Read the model definition and answer for the solid it produces. Units are mm, in the model's axes. Round coordinates to 2 decimals unless told otherwise and drop trailing zeros. Write each loop counter-clockwise with the first axis right and the second up, starting at its lowest first coordinate (ties: lowest second). Pieces come first, ordered by that corner, then holes. Notation, with made-up numbers: (57.25, 35) - (116.25, 35) arc R33 ccw to (116.25, 69) - close; hole circle Ø11 at (-8, 9.25). An arc over 180 degrees is marked (long way). Use one line per item in the form item = value. Start each with the question number.
1) The part is cut by section B-B, the plane z = 1. Give the vertices of the cut face in (x, y).
2) The part is cut by section A-A, the plane x = 53.5. Give the vertices of the cut face in (y, z), plus the area to 3 significant figures.
3) Consider line 1 along Y through (x, z) = (53, 0.4); line 2 along X through (y, z) = (18.5, 1.35); line 3 along Y through (x, z) = (14.5, 1.35). Determine where each line is inside the solid, lowest interval first. Write a range as from..to.
4) For a pull along Z with two mould halves and no side action, classify faces 1 (the face through (39, 10, 0)), 2 (the face through (39, 10, 1.5)) as released by +Z, released by -Z, zero draft, split by the parting line, or undercut.
5) This flat-tipped pin is pushed along its axis until it touches: pin 1 (2 mm diameter, centred on x = 71.5, y = 9, fed in from -Z). Where does it stop, or does it pass through?
from build123d import *

# Parameters (mm, degrees)
F0_W     = 80
F0_H     = 20
F1_DEPTH = 1.5
F2_SIZE  = 1.25
F3_R     = 0.5


with BuildPart() as f1:
    # F0 (on Top) → F1 (new body)
    with BuildSketch(Plane.XY):
        with Locations((40, 10)):
            Rectangle(F0_W, F0_H)
    extrude(amount=F1_DEPTH)

    # F2
    f2_edges = [f1.edges().sort_by_distance(p)[0] for p in [
        (0, 10, 1.5),
        (40, 0, 1.5),
        (80, 10, 1.5),
        (40, 20, 1.5),
    ]]
    chamfer(f2_edges, length=F2_SIZE)

    # F3
    f3_edges = [f1.edges().sort_by_distance(p)[0] for p in [
        (1.25, 10, 1.5),
        (40, 18.75, 1.5),
        (40, 1.25, 1.5),
        (78.75, 10, 1.5),
        (80, 10, 0.25),
        (40, 0, 0.25),
        (40, 20, 0.25),
        (0, 10, 0.25),
    ]]
    fillet(f3_edges, radius=F3_R)


solid = f1.part
Geometry results:
q1.outline = (0.75, 0.75) - (79.25, 0.75) - (79.25, 19.25) - (0.75, 19.25) - close
q2.outline = (0, 0) - (20, 0) - (20, 0.04) arc R0.5 ccw to (19.85, 0.4) - (18.9, 1.35) arc R0.5 ccw to (18.54, 1.5) - (1.46, 1.5) arc R0.5 ccw to (1.1, 1.35) - (0.15, 0.4) arc R0.5 ccw to (0, 0.04) - close
q2.area = 28.4 mm2
q3.line_1 = 0.15..19.85
q3.line_2 = 1.1..78.9
q3.line_3 = 1.1..18.9
q4.face_1 = released by -Z
q4.face_2 = released by +Z
q5.pin_1 = 0
